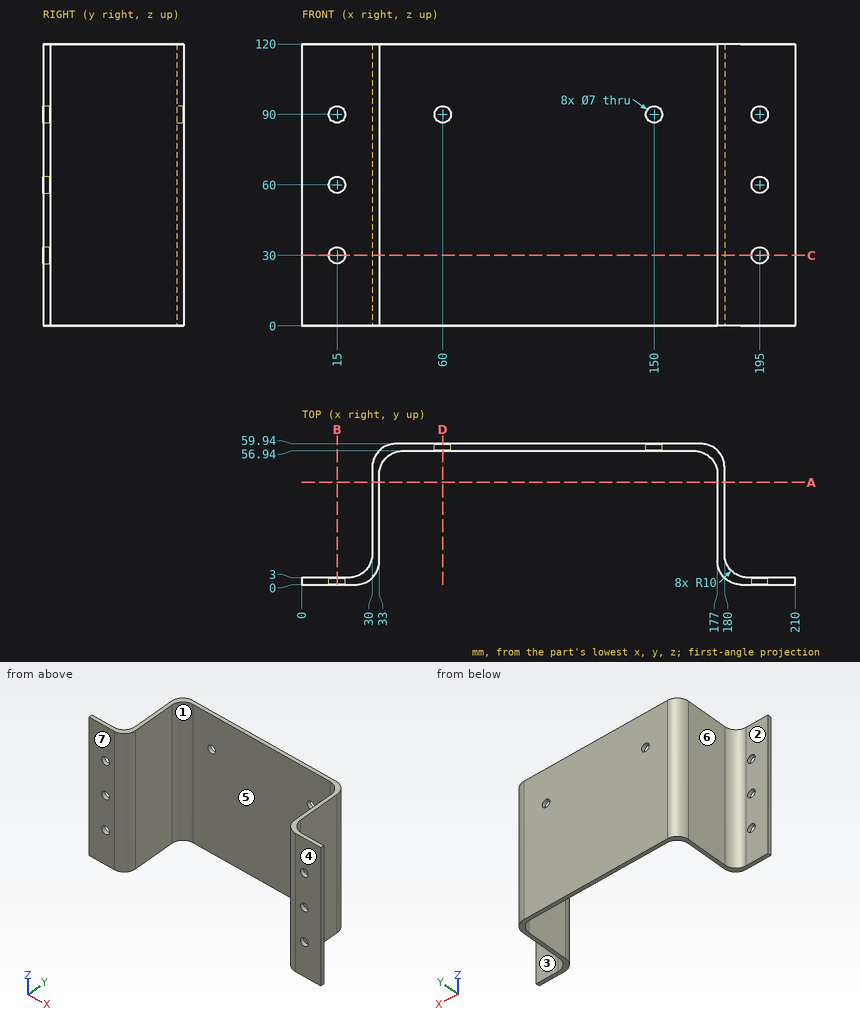
Part print with two shaded views. Sizes in mm from the minimum x, y, z corner. A direction names the side the tool comes from. Give positions to 0.01 mm unless a question says otherwise; leave off trailing zeros. Order: outer loops, then holes, each group sorted by start corner. A loop starts at its lowest first (then second) coordinate and runs counter-clockwise, first axis right, second up.
(1) Saw through at C-C, the plane z = 30. Give the cut face in (x, y), then the cut area to 3 significant figures.
(2) Saw through at A-A, the plane y = 43.5. Give the cut face in (x, z).
(3) Mould opens along X. For the marked faces 5, 6 and 7 say: released by +X, released by -X, zero draft, split by the parting line, or undercut.
(4) Saw through at D-D, the plane x = 60. Give the cut face in (y, z), then the cut area to 3 significant figures.
(5) Saw through at B-B, the plane x = 15. Give the cut face in (y, z).
(6) Drill centre lines: L1, parallel to Z at x = 15, y = 1.25; L2, parallel to X at y = 27.5, z = 105; L3, parallel to Z at x = 60, y = 59.05. Where is each one in solid material? Low to high.
(7) Flat gauge pins, fed straight in: pin 1 (10 mm diameter, centred on x = 125, z = 78.5, fed in from -Y); pin 2 (10 mm diameter, centred on x = 201, z = 75, fed in from +Y); pin 3 (4 mm diameter, centred on x = 60, z = 90, fed in from +Y); pin 4 (4 mm diameter, centred on y = 40.5, z = 90.5, fed in from -X). Where does each tip first touch, or does it go through?
(8) Tool access for the marked faces 1, 2, 3 and 4: list every direction of +Z, -Z, +X, -X, +Y, -Y with a clear straight run to the whole face (end or side of a thin tool).
Results found:
1. outline: (0, 0) - (11.5, 0) - (11.5, 3) - (0, 3) - close; (18.5, 0) - (23, 0) arc R10 ccw to (33, 10) - (33, 46.94) arc R10 cw to (43, 56.94) - (167, 56.94) arc R10 cw to (177, 46.94) - (177, 10) arc R10 ccw to (187, 0) - (191.5, 0) - (191.5, 3) - (190, 3) arc R10 cw to (180, 13) - (180, 49.94) arc R10 ccw to (170, 59.94) - (40, 59.94) arc R10 ccw to (30, 49.94) - (30, 13) arc R10 cw to (20, 3) - (18.5, 3) - close; (198.5, 0) - (210, 0) - (210, 3) - (198.5, 3) - close
1. area: 930 mm2
2. outline: (30, 0) - (33, 0) - (33, 120) - (30, 120) - close; (177, 0) - (180, 0) - (180, 120) - (177, 120) - close
3. face 5: undercut
3. face 6: released by -X
3. face 7: zero draft
4. outline: (56.94, 0) - (59.94, 0) - (59.94, 86.5) - (56.94, 86.5) - close; (56.94, 93.5) - (59.94, 93.5) - (59.94, 120) - (56.94, 120) - close
4. area: 339 mm2
5. outline: (0, 0) - (3, 0) - (3, 26.5) - (0, 26.5) - close; (0, 33.5) - (3, 33.5) - (3, 56.5) - (0, 56.5) - close; (0, 63.5) - (3, 63.5) - (3, 86.5) - (0, 86.5) - close; (0, 93.5) - (3, 93.5) - (3, 120) - (0, 120) - close
6. L1: z = 0 to 26.5, 33.5 to 56.5, 63.5 to 86.5, 93.5 to 120
6. L2: x = 30 to 33, 177 to 180
6. L3: z = 0 to 86.5, 93.5 to 120
7. pin 1: stops at y = 56.94
7. pin 2: stops at y = 3
7. pin 3: passes through
7. pin 4: stops at x = 30
8. face 1: +Z, -Z, -Y
8. face 2: +Z, -Z, -X, +Y
8. face 3: +Z, -Z, +X, +Y
8. face 4: +Z, -Z, +X, -X, -Y
